```python
from build123d import *

# Parameters (mm, degrees)
SKETCH_1_W      = 15
SKETCH_1_H      = 15
SKETCH_1_R      = 1.5
EXTRUDE_1_DEPTH = 5
SKETCH_2_W      = 15
SKETCH_2_H      = 15
SKETCH_2_R      = 1.5
EXTRUDE_2_DEPTH = 5


with BuildPart() as part:
    # 草图1 → 凸台-拉伸1 (new body)
    with BuildSketch(Plane(origin=(0, 0, 0), x_dir=(1, 0, 0), z_dir=(0, 1, 0))):
        with Locations((7.5, 7.5)):
            Rectangle(SKETCH_1_W, SKETCH_1_H)
        with Locations(Location((7.5, 10, 0), (0, 0, 270))):
            Circle(SKETCH_1_R, mode=Mode.SUBTRACT)
    extrude(amount=EXTRUDE_1_DEPTH)

    # 草图2 → 凸台-拉伸2 (add)
    with BuildSketch(Plane.XY):
        with Locations((7.5, 7.5)):
            Rectangle(SKETCH_2_W, SKETCH_2_H)
        with Locations((3, 10)):
            Circle(SKETCH_2_R, mode=Mode.SUBTRACT)
        with Locations((12, 10)):
            Circle(SKETCH_2_R, mode=Mode.SUBTRACT)
    extrude(amount=-EXTRUDE_2_DEPTH)


solid = part.part
```
Design review of the part built by this model. Coordinates are the model's own, in mm. A direction names the side the tool comes from. Round coordinates to 2 decimals unless told otherwise and drop trailing zeros. Write each loop counter-clockwise with the first axis right and the second up, starting at its lowest first coordinate (ties: lowest second). Pieces come first, ordered by that corner, then holes. Notation, with made-up numbers: (1, 23) -> (56, 23) arc R6 cw to (56, 32) -> close; hole circle Ø3 at (-28, 19). An arc over 180 degrees is marked (long way). Answer in a Markdown table with one row per item.
Q1. Take a section at A-A, the plane y = 10. State the section outline as (x, z) points.
The answers:
| item | result |
|---|---|
| outline | (0, -5) -> (1.5, -5) -> (1.5, 0) -> (0, 0) -> close; (4.5, -5) -> (10.5, -5) -> (10.5, 0) -> (4.5, 0) -> close; (13.5, -5) -> (15, -5) -> (15, 0) -> (13.5, 0) -> close |
Q2. Clearance check with flat-ended pins moving along their axes: pin 1 Ø2 at (x, z) = (5.5, -6.5) entering from +Y; pin 2 Ø3 at (x, y) = (6.5, 9.5) entering from -Z. State where each tip first meets the part, or that it passes through.
The answers:
| item | result |
|---|---|
| pin 1 | y = 5 |
| pin 2 | z = -5 |
Q3. Take a section at B-B, the plane z = -10. State the section outline as (x, y) points, then the cut area to 3 significant figures.
The answers:
| item | result |
|---|---|
| outline | (0, 0) -> (6, 0) -> (6, 5) -> (0, 5) -> close; (9, 0) -> (15, 0) -> (15, 5) -> (9, 5) -> close |
| area | 60.0 mm² |
Q4. Draft analysis for pull direction Z (two halves, no side actions). For faces 1 (the face through (10.8, 9.1, -2.5)), 2 (the face through (7, 7, 0)), 3 (the face through (7, 2, -15)), 4 (the face through (6, 2, -10)), state which applies: +Z half, -Z half, draft (parallel to the pull), parting line (faces both ways), or undercut.
The answers:
| item | result |
|---|---|
| face 1 | draft |
| face 2 | +Z half |
| face 3 | -Z half |
| face 4 | undercut |
Q5. For faces 5 (the face through (7, 0, -8)), 6 (the face through (5.7, 5, -10.1)), list the 3-axis set-ups (+Z, -Z, +X, -X, +Y, -Y) from which the entire face can be reached by the end or side of a thin tool; tool diameter is ignored.
The answers:
| item | result |
|---|---|
| face 5 | +Z, -Z, +X, -X, -Y |
| face 6 | -Z, +X, -X, +Y |
Q6. To check wall thickness, follow L1, parallel to X at y = 2.2, z = -10; L2, parallel to Y at x = 3, z = -3.4; L3, parallel to X at y = 9.5, z = -1. State the ranges of each line that lie inside material, in increasing order. Write a range as [from, to].
The answers:
| item | result |
|---|---|
| L1 | [0, 6], [9, 15] |
| L2 | [0, 8.5], [11.5, 15] |
| L3 | [0, 1.59], [4.41, 10.59], [13.41, 15] |
Q7. Take a section at D-D, the plane z = -1.75. State the section outline as (x, y) points, then the cut area to 3 significant figures.
The answers:
| item | result |
|---|---|
| outline | (0, 0) -> (15, 0) -> (15, 15) -> (0, 15) -> close; hole circle Ø3 at (3, 10); hole circle Ø3 at (12, 10) |
| area | 211 mm² |
Q8. Take a section at C-C, the plane x = 7.5. State the section outline as (y, z) points.
The answers:
| item | result |
|---|---|
| outline | (0, -15) -> (5, -15) -> (5, -11.5) -> (0, -11.5) -> close; (0, -8.5) -> (5, -8.5) -> (5, -5) -> (15, -5) -> (15, 0) -> (0, 0) -> close |
